Build history of the part. All positions in model axes, mm. A direction names the side the tool comes from. Round coordinates to 2 decimals unless told otherwise and drop trailing zeros. Write each loop counter-clockwise with the first axis right and the second up, starting at its lowest first coordinate (ties: lowest second). Pieces come first, ordered by that corner, then holes. Notation, with made-up numbers: M 24,-7 L 79,-7 A18 cw 79,17 Z; hole C 10,-12 d7. An arc over 180 degrees is marked long. One line per item, written item: value. Start each with the question number.
```python
from build123d import *

# Parameters (mm, degrees)
CUT_EXTRUDE_1_DEPTH = 0.6


with BuildPart() as part:
    # 草图1 → Revolve 651 (revolve)
    with BuildSketch(Plane.XY, mode=Mode.PRIVATE) as revolve_651_sk:
        with BuildLine():
            Line((0, 0), (0, 1.685882754))
            ThreePointArc((0, 1.685882754), (0.026272266, 1.753441774), (0.091284426, 1.785502223))
            Line((0.091284426, 1.785502223), (1.4, 1.9))
            Line((1.4, 1.9), (1.4, 1.05))
            ThreePointArc((1.4, 1.05), (1.429289322, 0.979289322), (1.5, 0.95))
            Line((1.5, 0.95), (2.11339746, 0.95))
            Line((2.11339746, 0.95), (2.2, 1))
            Line((2.2, 1), (31.4, 1))
            Line((31.4, 1), (31.4, 0))
            Line((31.4, 0), (0, 0))
        make_face()
    revolve(revolve_651_sk.sketch.rotate(Axis((0, 0, 0), (1, 0, 0)), 90), axis=Axis((0, 0, 0), (1, 0, 0)))

    # 草图2 → 切除-拉伸1 (cut)
    with BuildSketch(Plane.ZY):
        with BuildLine():
            Line((0.25, 1.88348082), (0.25, -1.88348082))
            ThreePointArc((0.25, -1.88348082), (0, -1.9), (-0.25, -1.88348082))
            Line((-0.25, -1.88348082), (-0.25, 1.88348082))
            ThreePointArc((-0.25, 1.88348082), (0, 1.9), (0.25, 1.88348082))
        make_face()
    extrude(amount=-CUT_EXTRUDE_1_DEPTH, mode=Mode.SUBTRACT)

    # 草图3 → 切除-旋转1 (revolve, cut)
    with BuildSketch(Plane(origin=(0, 0, 0), x_dir=(1, 0, 0), z_dir=(0, 1, 0)), mode=Mode.PRIVATE) as cut_revolve_1_sk:
        Polygon((31.200005867, 1), (31.599994133, 1), (31.4, 0.6536), align=None)
    revolve(cut_revolve_1_sk.sketch.rotate(Axis((0, 0, 0), (1, 0, 0)), 180), axis=Axis((0, 0, 0), (1, 0, 0)), mode=Mode.SUBTRACT)


solid = part.part
```
Item 1: Drill centre lines: line 1 (X direction, y = 0.95, z = -1.1); line 2 (X direction, y = 0.3, z = 0.2); line 3 (Z direction, x = 2.5, y = -0.05). Where is each one in solid material? Low to high.
Item 2: Cut at A-A, the plane y = 0. Write the cut outline in (x, z).
Item 3: Which spindle directions (+Z, -Z, +X, -X, +Y, -Y) get a long thin tool onto all of the face, cutting with end or side? Do faces 1 (the cylindrical face through (17, 1, 0)), 2 (the cylindrical face through (1.8, -0.3, 0.9)), 3 (the flat face through (0, 0, 1)). Say none if no direction does.
Item 4: Cut at B-B, the plane x = 20.5. Write the cut outline in (y, z), plus the area to 3 significant figures.
Item 5: Drop flat-ended pins along their axis: pin 1 (0.7 mm diameter, centred on x = 0.5, y = 0, fed in from +Z); pin 2 (1 mm diameter, centred on y = 1, z = 1, fed in from +X); pin 3 (1.5 mm diameter, centred on x = 4.5, z = 1, fed in from +Y). Give the stop position or say it passes through.
Computed values:
1. line 1: x = 0 to 1.4
1. line 2: x = 0.6 to 31.4
1. line 3: z = -1 to 1
2. outline: M 0,-1.69 A0.1 ccw 0.09,-1.79 L 1.4,-1.9 L 1.4,-1.05 A0.1 cw 1.5,-0.95 L 2.11,-0.95 L 2.2,-1 L 31.2,-1 L 31.4,-0.65 L 31.4,0.65 L 31.2,1 L 2.2,1 L 2.11,0.95 L 1.5,0.95 A0.1 cw 1.4,1.05 L 1.4,1.9 L 0.09,1.79 A0.1 ccw 0,1.69 L 0,0.25 L 0.6,0.25 L 0.6,-0.25 L 0,-0.25 Z
3. face 1: +X
3. face 2: none
3. face 3: +Z, -Z, -X, +Y, -Y
4. outline: C 0,0 d2
4. area: 3.14 mm2
5. pin 1: stops at z = 1.85
5. pin 2: stops at x = 31.25
5. pin 3: stops at y = 0.97
